```python
from build123d import *

# Parameters (mm, degrees)
F0_W     = 30
F0_H     = 50
F1_DEPTH = 5
F2_W     = 30
F2_H     = 15
F3_DEPTH = 5
F4_R     = 3.75
F5_DEPTH = 5.001
F6_R     = 10
F7_SIZE  = 1.25
F8_T     = -0.6


with BuildPart() as f1:
    # F0 (on Front) → F1 (new body)
    with BuildSketch(Plane.XZ):
        with Locations((15, 25)):
            Rectangle(F0_W, F0_H)
    extrude(amount=F1_DEPTH)

    # F2 (on face) → F3 (join)
    with BuildSketch(Plane.XZ.offset(5)):
        with Locations((15, 7.5)):
            Rectangle(F2_W, F2_H)
    extrude(amount=F3_DEPTH)

    # F4 (on face) → F5 (cut, through all)
    with BuildSketch(Plane.XZ.offset(5)):
        with Locations((10, 40)):
            Circle(F4_R)
    extrude(amount=-F5_DEPTH, mode=Mode.SUBTRACT)

    # F6
    f6_edges = [f1.edges().sort_by_distance(p)[0] for p in [
        (30, -2.5, 50),
        (30, -7.5, 15),
    ]]
    fillet(f6_edges, radius=F6_R)

    # F7
    f7_edges = [f1.edges().sort_by_distance(p)[0] for p in [
        (10, -5, 50),
        (10, -10, 15),
    ]]
    chamfer(f7_edges, length=F7_SIZE)

    # F8
    f8_openings = [f1.faces().sort_by_distance(p)[0] for p in [
        (14.961923, -4.988033, 0),
        (0, -3.637279, 20.90781),
        (14.962998, 0, 24.197378),
    ]]
    offset(amount=F8_T, openings=f8_openings, kind=Kind.INTERSECTION)


solid = f1.part
```
Here's how the part is built. I have some questions about the finished solid (model axes, mm). A direction names the side the tool comes from. Give positions to 0.01 mm unless a question says otherwise; leave off trailing zeros. Loops run counter-clockwise (first coordinate to the right, second up) from the corner with the lowest first, then second, coordinate; pieces in that order, holes last. Notation, with made-up numbers: M 18,60.25 L 56,60.25 A34 ccw 56,93.25 Z; hole C 88,89 d8. An arc over 180 degrees is marked long. Return JSON: item names as keys, results as strings.
Item 1: I'm going to push flat-ended pins straight in: pin 1 Ø8.5 at (x, z) = (9.5, 20) entering from +Y; pin 2 Ø4 at (x, y) = (6.5, -7.5) entering from +Z; pin 3 Ø14.5 at (x, z) = (16.5, 37.5) entering from -Y. Where does each tip first touch, or does it pass through?
A:
{"pin 1": "stops at y = -4.4", "pin 2": "stops at z = 15", "pin 3": "stops at y = -5"}
Item 2: On a 3-axis mill with a long thin cutter (end or side, diameter ignored), from which of +Z, -Z, +X, -X, +Y, -Y can I reach the whole of each face in a straight line? I mean faces 4 (the flat face through (10, -6, 14.4)), 5 (the cylindrical face through (9.434, -2.231, 44.313)), 6 (the flat face through (28.9, -4, 22.7)), 7 (the cylindrical face through (26.99, -6.84, 12.15)), 8 (the flat face through (10, -7, 15)). Say none if no direction works.
A:
{"face 4": "-Z, -X, +Y", "face 5": "+Y", "face 6": "-Z, +Y", "face 7": "+Z, +X, -Y", "face 8": "+Z, +X, -X, -Y"}
Item 3: Thinking about a two-plate mould opening in X: for faces 1 (the cylindrical face through (9.19, -2.54, 36.34)), 2 (the flat face through (29.37, -4.38, 22.74)), 3 (the flat face through (14, -5, 30)), which applies, released by +X, released by -X, zero draft, split by the parting line, or undercut?
A:
{"face 1": "undercut", "face 2": "released by +X", "face 3": "zero draft"}
Item 4: Imagine slicing it at B-B on z = 3. List the corners of the cut face in (x, y) for me.
A:
{"outline": "M 0,-10 L 28.75,-10 L 30,-8.75 L 30,0 L 29.4,0 L 29.4,-8.5 L 28.5,-9.4 L 0,-9.4 Z"}
Item 5: Imagine slicing it at C-C on x = 17.5. List the corners of the cut face in (y, z) for me.
A:
{"outline": "M -10,0 L -9.4,0 L -9.4,13.5 L -8.5,14.4 L -4.4,14.4 L -4.4,48.5 L -3.5,49.4 L 0,49.4 L 0,50 L -3.75,50 L -5,48.75 L -5,15 L -8.75,15 L -10,13.75 Z"}
Item 6: Imagine slicing it at A-A on x = 10. List the corners of the cut face in (y, z) for me, then the cut area to 3 significant figures.
A:
{"outline": "M -10,0 L -9.4,0 L -9.4,13.5 L -8.5,14.4 L -4.4,14.4 L -4.4,35.65 L 0,35.65 L 0,36.25 L -5,36.25 L -5,15 L -8.75,15 L -10,13.75 Z; M -5,43.75 L 0,43.75 L 0,44.35 L -4.4,44.35 L -4.4,48.5 L -3.5,49.4 L 0,49.4 L 0,50 L -3.75,50 L -5,48.75 Z", "area": "35.7 mm^2"}
Item 7: Imagine slicing it at D-D on z = 39.5. List the corners of the cut face in (x, y) for me, then the cut area to 3 significant figures.
A:
{"outline": "M 0,-5 L 6.28,-5 L 6.28,0 L 5.68,0 L 5.68,-4.4 L 0,-4.4 Z; M 13.72,-5 L 28.75,-5 L 30,-3.75 L 30,0 L 29.4,0 L 29.4,-3.5 L 28.5,-4.4 L 14.32,-4.4 L 14.32,0 L 13.72,0 Z", "area": "21.1 mm^2"}
Item 8: Please list where these lines run through material, in increasing order: line 1 (Z direction, x = 10, y = -2.85); line 2 (X direction, y = -1, z = 38); line 3 (Y direction, x = 20.5, z = 45.5).
A:
{"line 1": "z = 35.65 to 36.25, 43.75 to 44.35, 49.4 to 50", "line 2": "x = 6.14 to 6.83, 13.17 to 13.86, 29.4 to 30", "line 3": "y = -5 to -4.4"}
